from build123d import *

# Parameters (mm, degrees)
SKETCH1_R           = 1.5
SKETCH1_R_2         = 10
SKETCH1_R_3         = 22
SKETCH1_R_4         = 2.5
SKETCH1_R_5         = 12.5
BOSS_EXTRUDE1_DEPTH = 1


with BuildPart() as part:
    # Sketch1 → Boss-Extrude1 (new body)
    with BuildSketch(Plane(origin=(0, 0, 0), x_dir=(1, 0, 0), z_dir=(0, 1, 0))):
        with BuildLine():
            Line((92.071067812, 42.279220614), (42.279220614, 92.071067812))
            ThreePointArc((42.279220614, 92.071067812), (39.034987125, 94.238795325), (35.208152802, 95))
            Line((35.208152802, 95), (-35.208152802, 95))
            ThreePointArc((-35.208152802, 95), (-39.034987125, 94.238795325), (-42.279220614, 92.071067812))
            Line((-42.279220614, 92.071067812), (-92.071067812, 42.279220614))
            ThreePointArc((-92.071067812, 42.279220614), (-94.238795325, 39.034987125), (-95, 35.208152802))
            Line((-95, 35.208152802), (-95, -35.208152802))
            ThreePointArc((-95, -35.208152802), (-94.238795325, -39.034987125), (-92.071067812, -42.279220614))
            Line((-92.071067812, -42.279220614), (-42.279220614, -92.071067812))
            ThreePointArc((-42.279220614, -92.071067812), (-39.034987125, -94.238795325), (-35.208152802, -95))
            Line((-35.208152802, -95), (35.208152802, -95))
            ThreePointArc((35.208152802, -95), (39.034987125, -94.238795325), (42.279220614, -92.071067812))
            Line((42.279220614, -92.071067812), (92.071067812, -42.279220614))
            ThreePointArc((92.071067812, -42.279220614), (94.238795325, -39.034987125), (95, -35.208152802))
            Line((95, -35.208152802), (95, 35.208152802))
            ThreePointArc((95, 35.208152802), (94.238795325, 39.034987125), (92.071067812, 42.279220614))
        make_face()
        with Locations(Location((63.639610307, 63.639610307, 0), (0, 0, 270))):
            Circle(SKETCH1_R, mode=Mode.SUBTRACT)
        with Locations(Location((28.284271247, 28.284271247, 0), (0, 0, 270))):
            Circle(SKETCH1_R, mode=Mode.SUBTRACT)
        with Locations(Location((63.639610307, -63.639610307, 0), (0, 0, 270))):
            Circle(SKETCH1_R, mode=Mode.SUBTRACT)
        with Locations(Location((28.284271247, -28.284271247, 0), (0, 0, 270))):
            Circle(SKETCH1_R, mode=Mode.SUBTRACT)
        with Locations(Location((-63.639610307, -63.639610307, 0), (0, 0, 270))):
            Circle(SKETCH1_R, mode=Mode.SUBTRACT)
        with Locations(Location((-28.284271247, -28.284271247, 0), (0, 0, 270))):
            Circle(SKETCH1_R, mode=Mode.SUBTRACT)
        with Locations(Location((-63.639610307, 63.639610307, 0), (0, 0, 270))):
            Circle(SKETCH1_R, mode=Mode.SUBTRACT)
        with Locations(Location((-28.284271247, 28.284271247, 0), (0, 0, 270))):
            Circle(SKETCH1_R, mode=Mode.SUBTRACT)
        with Locations(Location((45.961940777, 45.961940777, 0), (0, 0, 270))):
            Circle(SKETCH1_R_2, mode=Mode.SUBTRACT)
        with Locations(Location((45.961940777, -45.961940777, 0), (0, 0, 270))):
            Circle(SKETCH1_R_2, mode=Mode.SUBTRACT)
        with Locations(Location((-45.961940777, -45.961940777, 0), (0, 0, 270))):
            Circle(SKETCH1_R_2, mode=Mode.SUBTRACT)
        with Locations(Location((0, 0, 0), (0, 0, 270))):
            Circle(SKETCH1_R_3, mode=Mode.SUBTRACT)
        with Locations(Location((32.5, 38.5, 0), (0, 0, 270))):
            Circle(SKETCH1_R_4, mode=Mode.SUBTRACT)
        with Locations(Location((89.5, 38.5, 0), (0, 0, 270))):
            Circle(SKETCH1_R_4, mode=Mode.SUBTRACT)
        with Locations(Location((32.5, -38.5, 0), (0, 0, 270))):
            Circle(SKETCH1_R_4, mode=Mode.SUBTRACT)
        with Locations(Location((89.5, -38.5, 0), (0, 0, 270))):
            Circle(SKETCH1_R_4, mode=Mode.SUBTRACT)
        with Locations(Location((-77.5, 0, 0), (0, 0, 270))):
            Circle(SKETCH1_R_5, mode=Mode.SUBTRACT)
        with Locations(Location((-45.961940777, 45.961940777, 0), (0, 0, 270))):
            Circle(SKETCH1_R_2, mode=Mode.SUBTRACT)
        with Locations(Location((-10.213834715, -90.213834715, 0), (0, 0, 270))):
            Circle(SKETCH1_R, mode=Mode.SUBTRACT)
        with Locations(Location((10.213834715, -69.786165285, 0), (0, 0, 270))):
            Circle(SKETCH1_R, mode=Mode.SUBTRACT)
        with Locations(Location((10.213834715, -90.213834715, 0), (0, 0, 270))):
            Circle(SKETCH1_R, mode=Mode.SUBTRACT)
        with Locations(Location((-10.213834715, -69.786165285, 0), (0, 0, 90))):
            Circle(SKETCH1_R, mode=Mode.SUBTRACT)
        with BuildLine():
            Line((27.079275596, 41.221411219), (16.142135624, 30.284271247))
            ThreePointArc((16.142135624, 30.284271247), (15.493288926, 29.850725745), (14.727922061, 29.69848481))
            Line((14.727922061, 29.69848481), (-14.727922061, 29.69848481))
            ThreePointArc((-14.727922061, 29.69848481), (-15.493288926, 29.850725745), (-16.142135624, 30.284271247))
            Line((-16.142135624, 30.284271247), (-27.079275596, 41.221411219))
            ThreePointArc((-27.079275596, 41.221411219), (-28.030817483, 42.551009763), (-28.502553799, 44.116490233))
            Line((-28.502553799, 44.116490233), (-32.40859259, 74.359545108))
            ThreePointArc((-32.40859259, 74.359545108), (-31.204928579, 78.301342571), (-27.449780482, 80))
            Line((-27.449780482, 80), (27.449780482, 80))
            ThreePointArc((27.449780482, 80), (31.204928579, 78.301342571), (32.40859259, 74.359545108))
            Line((32.40859259, 74.359545108), (28.502553799, 44.116490233))
            ThreePointArc((28.502553799, 44.116490233), (28.030817483, 42.551009763), (27.079275596, 41.221411219))
        make_face(mode=Mode.SUBTRACT)
        with BuildLine():
            Line((30.284271247, 16.142135624), (41.221411219, 27.079275596))
            ThreePointArc((41.221411219, 27.079275596), (42.551009763, 28.030817483), (44.116490233, 28.502553799))
            Line((44.116490233, 28.502553799), (74.359545108, 32.40859259))
            ThreePointArc((74.359545108, 32.40859259), (78.301342571, 31.204928579), (80, 27.449780482))
            Line((80, 27.449780482), (80, -27.449780482))
            ThreePointArc((80, -27.449780482), (78.301342571, -31.204928579), (74.359545108, -32.40859259))
            Line((74.359545108, -32.40859259), (44.116490233, -28.502553799))
            ThreePointArc((44.116490233, -28.502553799), (42.551009763, -28.030817483), (41.221411219, -27.079275596))
            Line((41.221411219, -27.079275596), (30.284271247, -16.142135624))
            ThreePointArc((30.284271247, -16.142135624), (29.850725745, -15.493288926), (29.69848481, -14.727922061))
            Line((29.69848481, -14.727922061), (29.69848481, 14.727922061))
            ThreePointArc((29.69848481, 14.727922061), (29.850725745, 15.493288926), (30.284271247, 16.142135624))
        make_face(mode=Mode.SUBTRACT)
        with BuildLine():
            Line((16.142135624, -30.284271247), (27.079275596, -41.221411219))
            ThreePointArc((27.079275596, -41.221411219), (28.030817483, -42.551009763), (28.502553799, -44.116490233))
            Line((28.502553799, -44.116490233), (32.40859259, -74.359545108))
            ThreePointArc((32.40859259, -74.359545108), (31.204928579, -78.301342571), (27.449780482, -80))
            Line((27.449780482, -80), (5.951214226, -80))
            ThreePointArc((5.951214226, -80), (5.027355519, -79.382733708), (5.24403049, -78.292970182))
            Line((5.24403049, -78.292970182), (6.875240199, -76.661405364))
            Line((6.875240199, -76.661405364), (11.981794054, -71.553739831))
            ThreePointArc((11.981794054, -71.553739831), (11.98140926, -68.018205946), (8.445875375, -68.01859074))
            Line((8.445875375, -68.01859074), (3.339706293, -73.125871458))
            Line((3.339706293, -73.125871458), (0.707183739, -75.758967125))
            ThreePointArc((0.707183739, -75.758967125), (0, -76.05193731), (-0.707183739, -75.758967125))
            Line((-0.707183739, -75.758967125), (-3.339706293, -73.125871458))
            Line((-3.339706293, -73.125871458), (-8.445875375, -68.01859074))
            ThreePointArc((-8.445875375, -68.01859074), (-11.98140926, -68.018205946), (-11.981794054, -71.553739831))
            Line((-11.981794054, -71.553739831), (-6.875240199, -76.661405364))
            Line((-6.875240199, -76.661405364), (-5.24403049, -78.292970182))
            ThreePointArc((-5.24403049, -78.292970182), (-5.027355519, -79.382733708), (-5.951214226, -80))
            Line((-5.951214226, -80), (-27.449780482, -80))
            ThreePointArc((-27.449780482, -80), (-31.204928579, -78.301342571), (-32.40859259, -74.359545108))
            Line((-32.40859259, -74.359545108), (-28.502553799, -44.116490233))
            ThreePointArc((-28.502553799, -44.116490233), (-28.030817483, -42.551009763), (-27.079275596, -41.221411219))
            Line((-27.079275596, -41.221411219), (-16.142135624, -30.284271247))
            ThreePointArc((-16.142135624, -30.284271247), (-15.493288926, -29.850725745), (-14.727922061, -29.69848481))
            Line((-14.727922061, -29.69848481), (14.727922061, -29.69848481))
            ThreePointArc((14.727922061, -29.69848481), (15.493288926, -29.850725745), (16.142135624, -30.284271247))
        make_face(mode=Mode.SUBTRACT)
        with BuildLine():
            Line((-30.284271247, -16.142135624), (-41.221411219, -27.079275596))
            ThreePointArc((-41.221411219, -27.079275596), (-42.551009763, -28.030817483), (-44.116490233, -28.502553799))
            Line((-44.116490233, -28.502553799), (-74.359545108, -32.40859259))
            ThreePointArc((-74.359545108, -32.40859259), (-78.301342571, -31.204928579), (-80, -27.449780482))
            Line((-80, -27.449780482), (-80, -19.5))
            ThreePointArc((-80, -19.5), (-79.414213562, -18.085786438), (-78, -17.5))
            Line((-78, -17.5), (-77.5, -17.5))
            ThreePointArc((-77.5, -17.5), (-60, 0), (-77.5, 17.5))
            Line((-77.5, 17.5), (-78, 17.5))
            ThreePointArc((-78, 17.5), (-79.414213562, 18.085786438), (-80, 19.5))
            Line((-80, 19.5), (-80, 27.449780482))
            ThreePointArc((-80, 27.449780482), (-78.301342571, 31.204928579), (-74.359545108, 32.40859259))
            Line((-74.359545108, 32.40859259), (-44.116490233, 28.502553799))
            ThreePointArc((-44.116490233, 28.502553799), (-42.551009763, 28.030817483), (-41.221411219, 27.079275596))
            Line((-41.221411219, 27.079275596), (-30.284271247, 16.142135624))
            ThreePointArc((-30.284271247, 16.142135624), (-29.850725745, 15.493288926), (-29.69848481, 14.727922061))
            Line((-29.69848481, 14.727922061), (-29.69848481, -14.727922061))
            ThreePointArc((-29.69848481, -14.727922061), (-29.850725745, -15.493288926), (-30.284271247, -16.142135624))
        make_face(mode=Mode.SUBTRACT)
    extrude(amount=BOSS_EXTRUDE1_DEPTH)


solid = part.part
Design review of the part built by this model. Coordinates are the model's own, in mm. A direction names the side the tool comes from. Round coordinates to 2 decimals unless told otherwise and drop trailing zeros. Loops run counter-clockwise (first coordinate to the right, second up) from the corner with the lowest first, then second, coordinate; pieces in that order, holes last. Notation, with made-up numbers: (44.5, 70.5) - (93.5, 70.5) arc R28 ccw to (93.5, 92.5) - close; hole circle Ø7 at (0, -5). An arc over 180 degrees is marked (long way). One line per item, written item: value. Start each with the question number.
1) Consider section A-A on x = 89.5. Give the boundary of the cut face in (y, z), then the cut area to 3 significant figures.
2) Insertion check: pin 1 Ø1.8 at (x, z) = (-28.28, -28.28) entering from +Y. The pin has a flat end and moves straight along its axis. Give the tip position at first contact, or say it passes through.
3) Consider section B-B on z = 50.5. Give the boundary of the cut face in (x, y).
4) For faces 1 (the flat face through (-1.3, 1, -22.4)), 2 (the cylindrical face through (78.26, 0.49, -31.24)), list the 3-axis set-ups (+Z, -Z, +X, -X, +Y, -Y) from which the entire face can be reached by the end or side of a thin tool; tool diameter is ignored.
5) Draft analysis for pull direction X (two halves, no side actions). For faces 3 (the cylindrical face through (34.61, 0.49, 39.84)), 4 (the cylindrical face through (-78.26, 0.49, 31.24)), 5 (the flat face through (-66.83, 0.49, -67.52)), 6 (the flat face through (-1.3, 0, -22.4)), state which applies: +X half, -X half, draft (parallel to the pull), parting line (faces both ways), or undercut.
6) Consider section C-C on z = -38.5. Give the boundary of the cut face in (x, y), then the cut area to 3 significant figures.
7) Consider section D-D on y = 0.8. Give the number of separate pieces and of enclosed holes in the cut face, then the cut area to 3 significant figures.
8) To check wall thickness, follow L1, parallel to X at y = 0.6, z = 0; L2, parallel to X at y = 0.8, z = 42.5; L3, parallel to Z at x = -22.5, y = 0.45. State the ranges of each line that lie inside material, in increasing order. Write a range as from..to.
Reported:
1. outline: (0, -44.85) - (1, -44.85) - (1, -41) - (0, -41) - close; (0, -36) - (1, -36) - (1, 36) - (0, 36) - close; (0, 41) - (1, 41) - (1, 44.85) - (0, 44.85) - close
1. area: 79.7 mm^2
2. pin 1: passes through
3. outline: (-83.85, 0) - (-54.87, 0) - (-54.87, 1) - (-83.85, 1) - close; (-37.05, 0) - (-29.33, 0) - (-29.33, 1) - (-37.05, 1) - close; (29.33, 0) - (37.05, 0) - (37.05, 1) - (29.33, 1) - close; (54.87, 0) - (83.85, 0) - (83.85, 1) - (54.87, 1) - close
4. face 1: +Z, -Z, +X, -X, +Y
4. face 2: +Y, -Y
5. face 3: undercut
5. face 4: undercut
5. face 5: -X half
5. face 6: draft
6. outline: (-94.44, 0) - (-52.62, 0) - (-52.62, 1) - (-94.44, 1) - close; (-39.3, 0) - (-24.36, 0) - (-24.36, 1) - (-39.3, 1) - close; (24.36, 0) - (30, 0) - (30, 1) - (24.36, 1) - close; (35, 0) - (39.3, 0) - (39.3, 1) - (35, 1) - close; (52.62, 0) - (87, 0) - (87, 1) - (52.62, 1) - close; (92, 0) - (94.44, 0) - (94.44, 1) - (92, 1) - close
6. area: 104 mm^2
7. separate pieces: 1
7. enclosed holes: 26
7. area: 15,800 mm^2
8. L1: x = -95..-90, -65..-60, -29.7..-22, 22..29.7, 80..95
8. L2: x = -91.85..-55.34, -36.58..-28.01, 28.01..36.58, 55.34..91.85
8. L3: z = -95..-80, -36.64..36.64, 80..95
